Read the model definition and answer for the solid it produces. Units are mm, in the model's axes. A direction names the side the tool comes from. Coordinates: 2 decimals unless noted, no trailing zeros. Order: outer loops, then holes, each group sorted by start corner. A loop starts at its lowest first (then second) coordinate and runs counter-clockwise, first axis right, second up.
Autodesk Inventor part; units mm, degrees
ref_plane "Work Plane1" through (0, 15.6, 3.5) normal (0, 1, 0) x (1, 0, 0)
ref_plane "YZ Plane" through (0, 0, 0) normal (1, 0, 0) x (0, 1, 0)
ref_plane "XZ Plane" through (0, 0, 0) normal (0, 1, 0) x (-1, 0, 0)
sketch "Sketch1" plane through (0, 0, 0) normal (0, 1, 0) x (-1, 0, 0)
  line L0 (-10, 16) -> (10, 16)
  line L1 (10, 16) -> (10, -16)
  line L2 (10, -16) -> (-10, -16)
  line L3 (-10, -16) -> (-10, 16)
  line L4 (-10, 16) -> (10, -16) construction
  line L5 (10, 16) -> (-10, -16) construction
  point P0 (0, 0)
  dimension "d0" = 20
  dimension "d1" = 32
extrude "Extrusion1" add sketch "Sketch1" along normal blind 1.6
sketch "Sketch3" plane through (0, 1.6, 0) normal (0, 1, 0) x (1, 0, 0)
  line L0 (-10, 16) -> (-10, -16)
  line L1 (-10, -16) -> (-7.5, -16)
  line L2 (-10, -16) -> (10, -16)
  line L3 (-7.5, -16) -> (-7.5, -13.5)
  circle A0 centre (-7.5, -13.5) radius 1.5
  point P0 (0, 0)
  dimension "d4" = 2.5
  dimension "d5" = 2.5
  dimension "d6" = 3
extrude "Extrusion2" cut sketch "Sketch3" against normal blind 1.6
pattern_linear "Rectangular Pattern1" count 2 spacing 27 along (0, 0, -1) count 2 spacing 15 along (1, 0, 0) of "Extrusion2"
sketch "Sketch4" plane through (0, 1.6, 0) normal (0, 1, 0) x (1, 0, 0)
  line L0 (-10, -16) -> (10, -16)
  line L1 (10, 16) -> (-10, 16)
  circle A0 centre (0, -3.5) radius 9.5
  point P0 (0, 0)
extrude "Extrusion3" add sketch "Sketch4" along normal blind 5
ref_plane "Work Plane1" through (0, 15.6, 3.5) normal (0, 1, 0) x (1, 0, 0)
sketch "Sketch5" plane through (0, 15.6, 3.5) normal (0, 1, 0) x (1, 0, 0)
  circle A0 centre (0, 0) radius 6.3
  point P0 (0, 3.5)
  dimension "d22" = 12.6
sketch "Sketch6" plane through (0, 6.6, 3.5) normal (0, 1, 0) x (1, 0, 0)
  circle A0 centre (0, 0) radius 9.5
  point P0 (0, 3.5)
loft "Loft1" add profiles "Sketch5" section 1 edges at (-9.5, 6.6, 3.5)
sketch "Sketch7" plane through (0, 0, 0) normal (0, -1, 0) x (1, 0, 0)
  line L0 (9.9296, -16.0477) -> (10, -10.0481)
  line L1 (10, 16) -> (10, -16)
  line L2 (10, -10.0481) -> (3, -10.0481)
  line L3 (3, -10.0481) -> (3, -3.1481)
  line L4 (3, -3.1481) -> (10, -3.1481)
  line L5 (10, -3.1481) -> (10, -10.0481)
  point P0 (0, 0)
  dimension "d27" = 6
  dimension "d28" = 7
  dimension "d29" = 6.9
extrude "Extrusion4" add sketch "Sketch7" along normal blind 5.3
properties part number "SensorGas"
Q1. The part is cut by section D-D, the plane y = 5.5. Determine the outline of the cut face in (x, z), then the cut area to 3 significant figures.
Q2. The part is cut by section A-A, the plane z = 13.5. Determine the outline of the cut face in (x, y), then the cut area to 3 significant figures.
Q3. Straight lines are drawn through the part: L1, parallel to Z at x = 7.5, y = 0.4; L2, parallel to X at y = 1.1, z = 13.5; L3, parallel to Y at x = -7.5, z = -9. For each, find the intervals that lie inside material, in ascending order.
Q4. Which of the six approach directions +Z, -Z, +X, -X, +Y, -Y give full straight-line access (tool end or side, diameter ignored) to faces 4 (the flat face through (3, -3, -7)), 5 (the cylindrical face through (5.11, 4.06, 11.51)), 6 (the flat face through (6, -3, -3.148)), 7 (the flat face through (10, 0, -4)), 8 (the cylindrical face through (-9, 0.81, 13.43))?
Q5. The part is cut by section C-C, the plane z = -6.5. Determine the outline of the cut face in (x, y).
Q6. Determine the mould class of faces 1 (the flat face through (7, -3, -10.048)), 2 (the flat face through (-10, 1, 0)), 3 (the cylindrical face through (6.3, 0.8, -12.6)) for opening direction X: +X half, -X half, draft (parallel to the pull), parting line (faces both ways), or undercut.
Q7. Each of these flat-tipped pins is pushed along its axis until it touches: P1, Ø1.6, axis at y = -1.5, z = -8, coming from the -X side; P2, Ø12, axis at x = -2, y = 8.5, coming from the -Z side; P3, Ø3, axis at x = -6.5, z = -10.5, coming from the +Y side; P4, Ø2.5, axis at x = 7.5, z = -13.5, coming from the +Y side. Where does it stop, or does it pass through?
Q8. The part is cut by section B-B, the plane x = 0. Determine the outline of the cut face in (y, z), then the cut area to 3 significant figures.
Computed values:
1. outline: circle Ø19 at (0, 3.5)
1. area: 284 mm2
2. outline: (-10, 0) - (-9, 0) - (-9, 1.6) - (-10, 1.6) - close; (-6, 0) - (6, 0) - (6, 1.6) - (-6, 1.6) - close; (9, 0) - (10, 0) - (10, 1.6) - (9, 1.6) - close
2. area: 22.4 mm2
3. L1: z = -16 to -15, -12 to 12, 15 to 16
3. L2: x = -10 to -9, -6 to 6, 9 to 10
3. L3: y = 0 to 1.6
4. face 4: +Z, -Z, -X, -Y
4. face 5: +Y
4. face 6: +Z, +X, -X, -Y
4. face 7: +Z, -Z, +X, +Y, -Y
4. face 8: +Y, -Y
5. outline: (-10, 0) - (3, 0) - (3, -5.3) - (10, -5.3) - (10, 1.6) - (-10, 1.6) - close
6. face 1: draft
6. face 2: -X half
6. face 3: undercut
7. P1: stops at x = 3
7. P2: stops at z = -6
7. P3: stops at y = 1.6
7. P4: passes through
8. outline: (0, -16) - (1.6, -16) - (1.6, -6) - (6.6, -6) - (15.6, -2.8) - (15.6, 9.8) - (6.6, 13) - (1.6, 13) - (1.6, 16) - (0, 16) - close
8. area: 288 mm2
